Check sheet for the drawn part. Datum: minimum x, y, z corner. Units: mm. A direction names the side the tool comes from. Coordinates: 2 decimals unless noted, no trailing zeros. Write each loop counter-clockwise with the first axis right and the second up, starting at its lowest first coordinate (ties: lowest second). Pieces come first, ordered by that corner, then holes. Notation, with made-up numbers: (-13.5, 67) - (9.5, 67) arc R24 ccw to (9.5, 104) - close; hole circle Ø10 at (-34.5, -39.75). An arc over 180 degrees is marked (long way). Use one line per item in the form item = value. Start each with the question number.
1. Cross-section at C-C on z = 4.1. Record the boundary of the cut face in (x, y).
2. Scan lines: line 1 along Y through (x, z) = (40, 3.1); line 2 along X through (y, z) = (7.5, 2.15); line 3 along X through (y, z) = (20, 3.5). Record each from-to range of solid material in increasing order.
3. Tool access check on the marked faces 1 and 2. Record the directions out of +Z, -Z, +X, -X, +Y, -Y that give a thin tool (end or side, any length) a straight path to the whole face; none if there is none.
4. Cross-section at A-A on y = 7.5. Record the boundary of the cut face in (x, z).
5. Cross-section at B-B on x = 10. Record the boundary of the cut face in (y, z), then the cut area to 3 significant figures.
6. Go/stop test with a flat-tipped pin: pin 1 Ø11 at (x, y) = (33, 21) entering from -Z. Record where the tip stops, or that it passes through.
7. Cross-section at D-D on z = 1.35. Record the boundary of the cut face in (x, y), then the cut area to 3 significant figures.
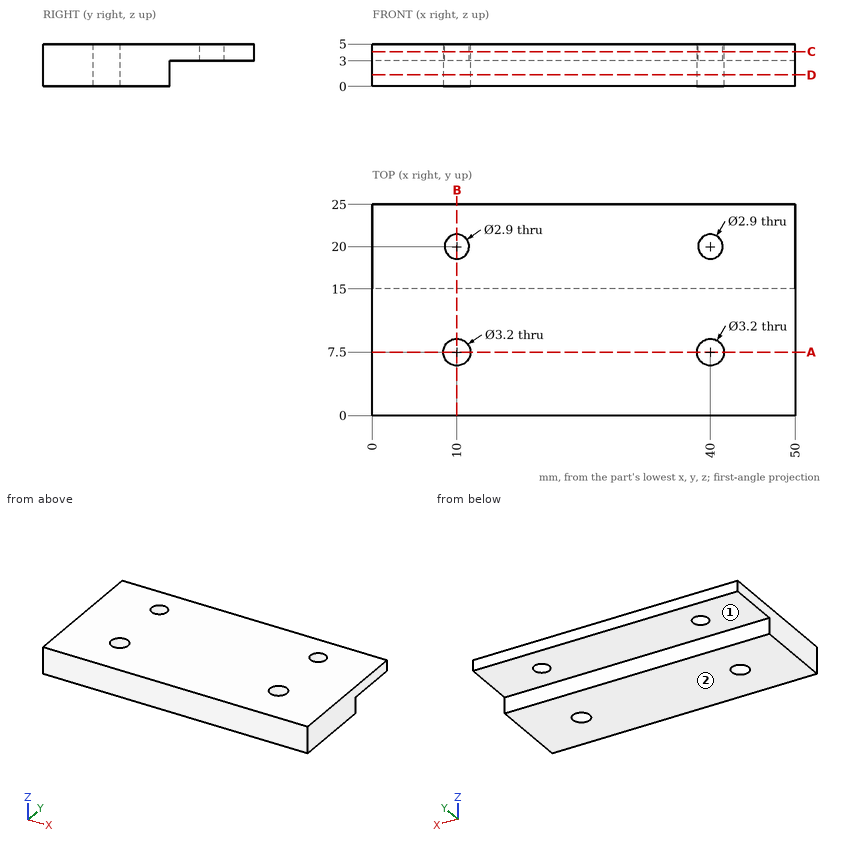
Final values:
q1.outline = (0, 0) - (50, 0) - (50, 25) - (0, 25) - close; hole circle Ø3.2 at (10, 7.5); hole circle Ø2.9 at (10, 20); hole circle Ø3.2 at (40, 7.5); hole circle Ø2.9 at (40, 20)
q2.line_1 = 0 to 5.9, 9.1 to 18.55, 21.45 to 25
q2.line_2 = 0 to 8.4, 11.6 to 38.4, 41.6 to 50
q2.line_3 = 0 to 8.55, 11.45 to 38.55, 41.45 to 50
q3.face_1 = -Z, +X, -X, +Y
q3.face_2 = -Z, +X, -X, +Y, -Y
q4.outline = (0, 0) - (8.4, 0) - (8.4, 5) - (0, 5) - close; (11.6, 0) - (38.4, 0) - (38.4, 5) - (11.6, 5) - close; (41.6, 0) - (50, 0) - (50, 5) - (41.6, 5) - close
q5.outline = (0, 0) - (5.9, 0) - (5.9, 5) - (0, 5) - close; (9.1, 0) - (15, 0) - (15, 3) - (18.55, 3) - (18.55, 5) - (9.1, 5) - close; (21.45, 3) - (25, 3) - (25, 5) - (21.45, 5) - close
q5.area = 73.2 mm²
q6.pin_1 = 3
q7.outline = (0, 0) - (50, 0) - (50, 15) - (0, 15) - close; hole circle Ø3.2 at (10, 7.5); hole circle Ø3.2 at (40, 7.5)
q7.area = 734 mm²
